```python
from build123d import *

# Parameters (mm, degrees)
SKETCH1_R           = 2
SKETCH1_R_2         = 12.6
SKETCH1_R_3         = 1.5
BOSS_EXTRUDE1_DEPTH = 5


with BuildPart() as part:
    # Sketch1 → Boss-Extrude1 (new body)
    with BuildSketch(Plane(origin=(0, 0, 0), x_dir=(1, 0, 0), z_dir=(0, 1, 0))):
        with BuildLine():
            Line((-0.695602201, -26.001013021), (19.342742394, -26.333158484))
            ThreePointArc((19.342742394, -26.333158484), (20.605232337, -25.984002388), (21.476990945, -25.006337943))
            Line((21.476990945, -25.006337943), (27.115129107, 4.255894982))
            ThreePointArc((27.115129107, 4.255894982), (26.312930803, 7.784075148), (25.748803556, 11.35805582))
            Line((25.748803556, 11.35805582), (19.484079103, 28.225152951))
            ThreePointArc((19.484079103, 28.225152951), (18.652270353, 29.305251267), (17.355348812, 29.725385394))
            Line((17.355348812, 29.725385394), (-14.839037586, 28.440806231))
            ThreePointArc((-14.839037586, 28.440806231), (-16.054862276, 28.031135004), (-16.861770169, 27.033658807))
            Line((-16.861770169, 27.033658807), (-24.050617364, 9.90476375))
            ThreePointArc((-24.050617364, 9.90476375), (-21.803670495, -14.182259815), (-0.695602201, -26.001013021))
        make_face()
        with Locations(Location((0, 19.5, 0), (0, 0, 270))):
            Circle(SKETCH1_R, mode=Mode.SUBTRACT)
        with Locations(Location((19.5, 0, 0), (0, 0, 270))):
            Circle(SKETCH1_R, mode=Mode.SUBTRACT)
        with Locations(Location((0, -19.5, 0), (0, 0, 270))):
            Circle(SKETCH1_R, mode=Mode.SUBTRACT)
        with Locations(Location((-19.5, 0, 0), (0, 0, 270))):
            Circle(SKETCH1_R, mode=Mode.SUBTRACT)
        with Locations(Location((0, 0, 0), (0, 0, 270))):
            Circle(SKETCH1_R_2, mode=Mode.SUBTRACT)
        with Locations(Location((19.381166369, -24.015039037, 0), (0, 0, 270))):
            Circle(SKETCH1_R_3, mode=Mode.SUBTRACT)
        with Locations(Location((17.326233239, 27.42369259, 0), (0, 0, 270))):
            Circle(SKETCH1_R_3, mode=Mode.SUBTRACT)
        with Locations(Location((-14.742076054, 26.144041757, 0), (0, 0, 270))):
            Circle(SKETCH1_R_3, mode=Mode.SUBTRACT)
    extrude(amount=BOSS_EXTRUDE1_DEPTH)


solid = part.part
```
For this review, take the finished solid that the model builds, in its own axes (mm). Round coordinates to 2 decimals unless told otherwise and drop trailing zeros. Order: outer loops, then holes, each group sorted by start corner. A loop starts at its lowest first (then second) coordinate and runs counter-clockwise, first axis right, second up.
Q1. Insertion check: P1, Ø2.5, axis at x = 17.33, z = -27.42, coming from the -Y side; P2, Ø1.5, axis at y = 3, z = 19.5, coming from the +X side. Each pin has a flat end and moves straight along its axis. Give the tip position at first contact, or say it passes through.
Findings below:
P1: passes through
P2: stops at x = 22.68
Q2. Mouldability with a two-part tool opening along X and no side actions: class faces 1 (the flat face through (22.66, 2.46, -19.67)), 2 (the cylindrical face through (-7.667, 2.465, -9.999)), 3 (the flat face through (12, 5, -8)), 4 (the cylindrical face through (-1.774, 2.465, -18.577)) as pulls with the +X half, pulls with the -X half, needs draft (parallel to the pull), parting line crosses it, or undercut.
Findings below:
face 1: pulls with the +X half
face 2: undercut
face 3: needs draft
face 4: undercut
Q3. We need section A-A, the plane z = -19.5. Give the boundary of the cut face in (x, y), plus the area to 3 significant figures.
Findings below:
outline: (-20.02, 0) - (-2, 0) - (-2, 5) - (-20.02, 5) - close; (2, 0) - (22.72, 0) - (22.72, 5) - (2, 5) - close
area: 194 mm2
Q4. We need section B-B, the plane y = 2.3. State how many separate pieces and enclosed holes the cut face has, plus the area to 3 significant figures.
Findings below:
separate pieces: 1
enclosed holes: 8
area: 1,920 mm2
Q5. Wall thickness on line 1 (X direction, y = 2.85, z = 0); line 2 (Z direction, x = -0.5, y = 0.35); line 3 (X direction, y = 4.2, z = -27): over which ranges is each line inside the solid? List them lowest first.
Findings below:
line 1: x = -26.01 to -21.5, -17.5 to -12.6, 12.6 to 17.5, 21.5 to 26.3
line 2: z = -29.01 to -21.44, -17.56 to -12.59, 12.59 to 17.56, 21.44 to 26
line 3: x = -16.88 to -15.97, -13.51 to 15.89, 18.77 to 19.94
Q6. We need section D-D, the plane x = 0. Give the boundary of the cut face in (y, z).
Findings below:
outline: (0, -29.03) - (5, -29.03) - (5, -21.5) - (0, -21.5) - close; (0, -17.5) - (5, -17.5) - (5, -12.6) - (0, -12.6) - close; (0, 12.6) - (5, 12.6) - (5, 17.5) - (0, 17.5) - close; (0, 21.5) - (5, 21.5) - (5, 26.01) - (0, 26.01) - close
Q7. We need section C-C, the plane z = -1. Give the boundary of the cut face in (x, y).
Findings below:
outline: (-25.99, 0) - (-21.23, 0) - (-21.23, 5) - (-25.99, 5) - close; (-17.77, 0) - (-12.56, 0) - (-12.56, 5) - (-17.77, 5) - close; (12.56, 0) - (17.77, 0) - (17.77, 5) - (12.56, 5) - close; (21.23, 0) - (26.49, 0) - (26.49, 5) - (21.23, 5) - close
